Drawing for the job (mm, zero at the part's lowest x, y, z). A direction names the side the tool comes from. Give positions to 0.01 mm unless a question says otherwise; leave off trailing zeros. Order: outer loops, then holes, each group sorted by start corner. A loop starts at its lowest first (then second) coordinate and runs counter-clockwise, first axis right, second up. Notation, with made-up numbers: M 68,-35.75 L 120,-35.75 A25 cw 120,-21.75 Z; hole C -20.5,13.25 d1. An arc over 180 degrees is marked long. One line per item, written item: value.
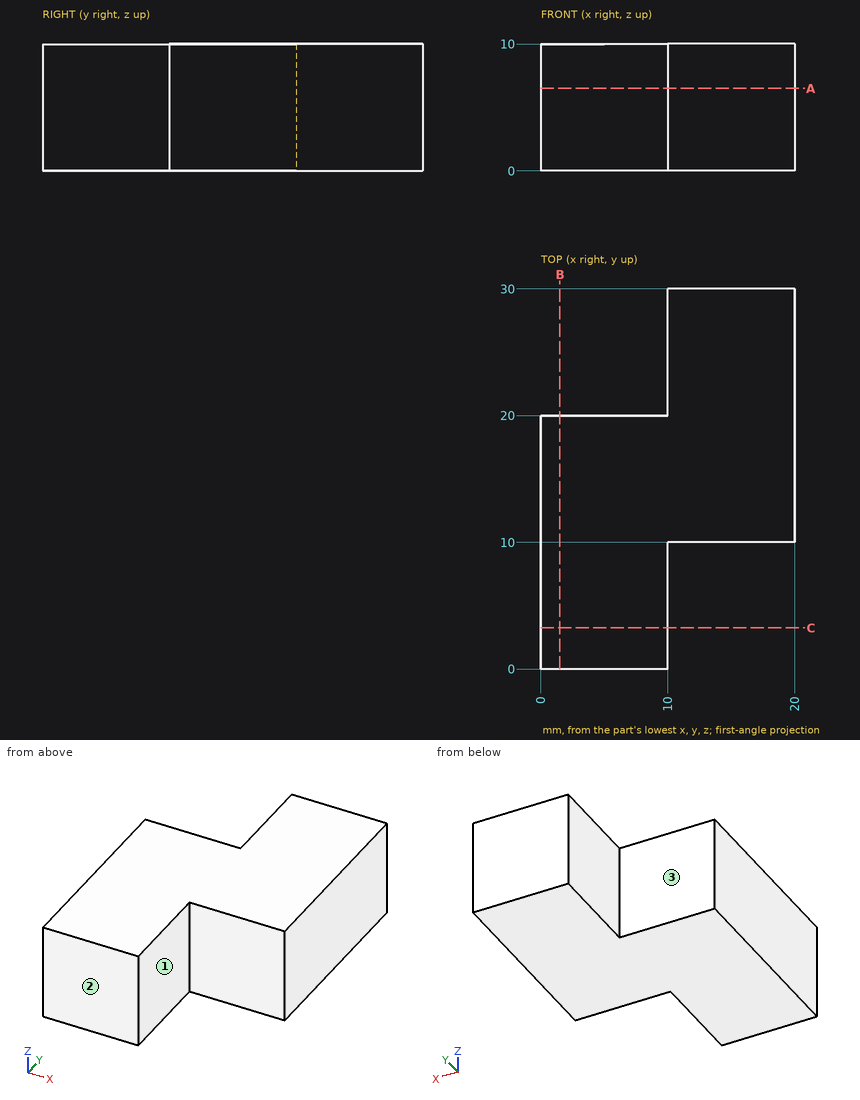
1) Saw through at A-A, the plane z = 6.5. Write the cut outline in (x, y), then the cut area to 3 significant figures.
Check values:
outline: M 0,0 L 10,0 L 10,10 L 20,10 L 20,30 L 10,30 L 10,20 L 0,20 Z
area: 400 mm^2
2) Pin check, flat tips, straight feed: pin 1 (5 mm diameter, centred on x = 13, z = 6, fed in from -Y); pin 2 (4 mm diameter, centred on y = 7, z = 2.5, fed in from +X); pin 3 (4 mm diameter, centred on y = 26.5, z = 8, fed in from -X). Stop position of each tip, or through.
Check values:
pin 1: y = 10
pin 2: x = 10
pin 3: x = 10
3) Saw through at C-C, the plane y = 3.25. Write the cut outline in (x, z).
Check values:
outline: M 0,0 L 10,0 L 10,10 L 0,10 Z
4) Saw through at B-B, the plane x = 1.5. Write the cut outline in (y, z), then the cut area to 3 significant figures.
Check values:
outline: M 0,0 L 20,0 L 20,10 L 0,10 Z
area: 200 mm^2
5) Drill centre lines: probe 1 along X at (y, z) = (22.75, 8.75); probe 2 along Y at (x, z) = (10.75, 2.75); probe 3 along X at (y, z) = (4.75, 7.5). Where is each one in solid material? Low to high. Write a range as from..to.
Check values:
probe 1: 10..20
probe 2: 10..30
probe 3: 0..10
6) Tool access for the marked faces 1, 2 and 3: list every direction of +Z, -Z, +X, -X, +Y, -Y with a clear straight run to the whole face (end or side of a thin tool).
Check values:
face 1: +Z, -Z, +X, -Y
face 2: +Z, -Z, +X, -X, -Y
face 3: +Z, -Z, -X, +Y
